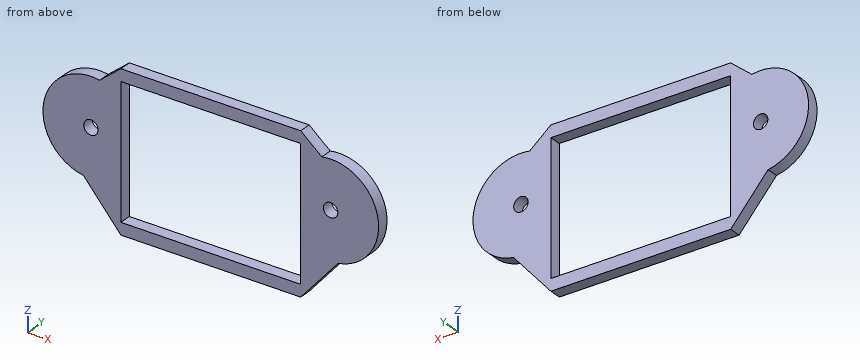
Autodesk Inventor part; units mm, degrees
ref_plane "YZ Plane" through (0, 0, 0) normal (1, 0, 0) x (0, 1, 0)
ref_plane "XZ Plane" through (0, 0, 0) normal (0, 1, 0) x (-1, 0, 0)
ref_plane "XY Plane" through (0, 0, 0) normal (0, 0, 1) x (1, 0, 0)
sketch "Esquisse1" plane through (0, 0, 0) normal (0, 1, 0) x (-1, 0, 0)
  line L0 (-37.5, 22) -> (37.5, 22)
  line L1 (37.5, 22) -> (37.5, -33)
  line L2 (37.5, -33) -> (-37.5, -33)
  line L3 (-37.5, -33) -> (-37.5, 22)
  line L4 (-37.5, 22) -> (37.5, 22)
  line L5 (37.5, 22) -> (37.5, 27)
  line L6 (37.5, 27) -> (-37.5, 27)
  line L7 (-37.5, 27) -> (-37.5, 22)
  line L8 (37.5, -33) -> (-37.5, -33)
  line L9 (-37.5, -33) -> (-37.5, -38)
  line L10 (-37.5, -38) -> (37.5, -38)
  line L11 (37.5, -38) -> (37.5, -33)
  circle A0 centre (-50, 0) radius 3
  arc A1 (-37.5, 15.6125) -> (-37.5, -15.6125) centre (-50, 0) ccw
  circle A2 centre (50, 0) radius 3
  arc A3 (37.5, -15.6125) -> (37.5, 15.6125) centre (50, 0) ccw
  line L12 (0, 0) -> (124.0045, 0) construction
  line L13 (-37.5, 27) -> (-70, 0)
  line L14 (-70, 0) -> (-37.5, -38)
  line L15 (37.5, 27) -> (70, 0)
  line L16 (37.5, -38) -> (70, 0)
  arc A4 (-37.5, -15.6125) -> (-37.5, 15.6125) centre (-50, 0) ccw
  arc A5 (30, 0) -> (37.5, -15.6125) centre (50, 0) ccw
  arc A6 (37.5, 15.6125) -> (30, 0) centre (50, 0) ccw
  dimension "d0" = 6
  dimension "d1" = 6
  dimension "d2" = 40
  dimension "d3" = 40
  dimension "d4" = 75
  dimension "d5" = 37.5
  dimension "d6" = 22
  dimension "d7" = 55
  dimension "d8" = 5
  dimension "d9" = 5
  dimension "d10" = 100
  dimension "d11" = 50
extrude "Extrusion1" add sketch "Esquisse1" along normal blind 5 contours L7 L6 L5 L0 | L3 A1 L13 L7 | L5 L15 A3 L1 | L3 A1 L14 L13 | A3 L15 L16 L1 | L3 L9 L14 A1 | L13 A1 | A3 L16 L11 L1 | A3 L15 | L2 L11 L10 L9 | A1 L14 | L16 A3
equation "\"d5\" = 0.5 * d4"
equation "\"d9\" = d8"
equation "\"d11\" = 0.5 * d10"
properties part number "support_batteries"
The listing builds one solid part. Answer for the finished solid, in the listing's coordinates (mm). Round coordinates to 2 decimals unless told otherwise and drop trailing zeros. Order: outer loops, then holes, each group sorted by start corner. A loop starts at its lowest first (then second) coordinate and runs counter-clockwise, first axis right, second up. Notation, with made-up numbers: (-15.5, 80) -> (-9.5, 80) arc R10 ccw to (-9.5, 88) -> close; hole circle Ø5 at (47, 76). An arc over 180 degrees is marked (long way). Put each result on its own line as item: value.
Q1. Consider line 1 along Z through (x, y) = (-15.5, 4.4); line 2 along X through (y, z) = (2.7, -1.5); line 3 along X through (y, z) = (4.7, 6). Determine where each line is inside the solid, lowest interval first.
Results list:
line 1: -38 to -33, 22 to 27
line 2: -69.94 to -52.6, -47.4 to -37.5, 37.5 to 47.4, 52.6 to 69.94
line 3: -69.08 to -37.5, 37.5 to 69.08
Q2. Section B-B, the plane z = 0 is taken. Write down the section's boundary in (x, y), and give its area (3 significant figures).
Results list:
outline: (-70, 0) -> (-53, 0) -> (-53, 5) -> (-70, 5) -> close; (-47, 0) -> (-37.5, 0) -> (-37.5, 5) -> (-47, 5) -> close; (37.5, 0) -> (47, 0) -> (47, 5) -> (37.5, 5) -> close; (53, 0) -> (70, 0) -> (70, 5) -> (53, 5) -> close
area: 265 mm^2
Q3. This flat-tipped pin is pushed along its axis until it touches: P1, Ø3, axis at y = 2.5, z = -4, coming from the -X side. Where does it stop, or does it pass through?
Results list:
P1: x = -69.84
Q4. Section C-C, the plane y = 2.2 is taken. Write down the section's boundary in (x, z), and give its area (3 significant figures).
Results list:
outline: (-53.1, -19.76) -> (-37.5, -38) -> (37.5, -38) -> (53.1, -19.76) arc R20 ccw (long way) to (46.33, 19.66) -> (37.5, 27) -> (-37.5, 27) -> (-46.33, 19.66) arc R20 ccw (long way) to start; hole circle Ø6 at (-50, 0); hole (-37.5, -33) -> (37.5, -33) -> (37.5, 22) -> (-37.5, 22) -> close; hole circle Ø6 at (50, 0)
area: 3,290 mm^2
Q5. Section D-D, the plane z = -17 is taken. Write down the section's boundary in (x, y), and give its area (3 significant figures).
Results list:
outline: (-60.54, 0) -> (-37.5, 0) -> (-37.5, 5) -> (-60.54, 5) -> close; (37.5, 0) -> (60.54, 0) -> (60.54, 5) -> (37.5, 5) -> close
area: 230 mm^2
Q6. Section A-A, the plane x = 7 is taken. Write down the section's boundary in (y, z), and give its area (3 significant figures).
Results list:
outline: (0, -38) -> (5, -38) -> (5, -33) -> (0, -33) -> close; (0, 22) -> (5, 22) -> (5, 27) -> (0, 27) -> close
area: 50.0 mm^2
